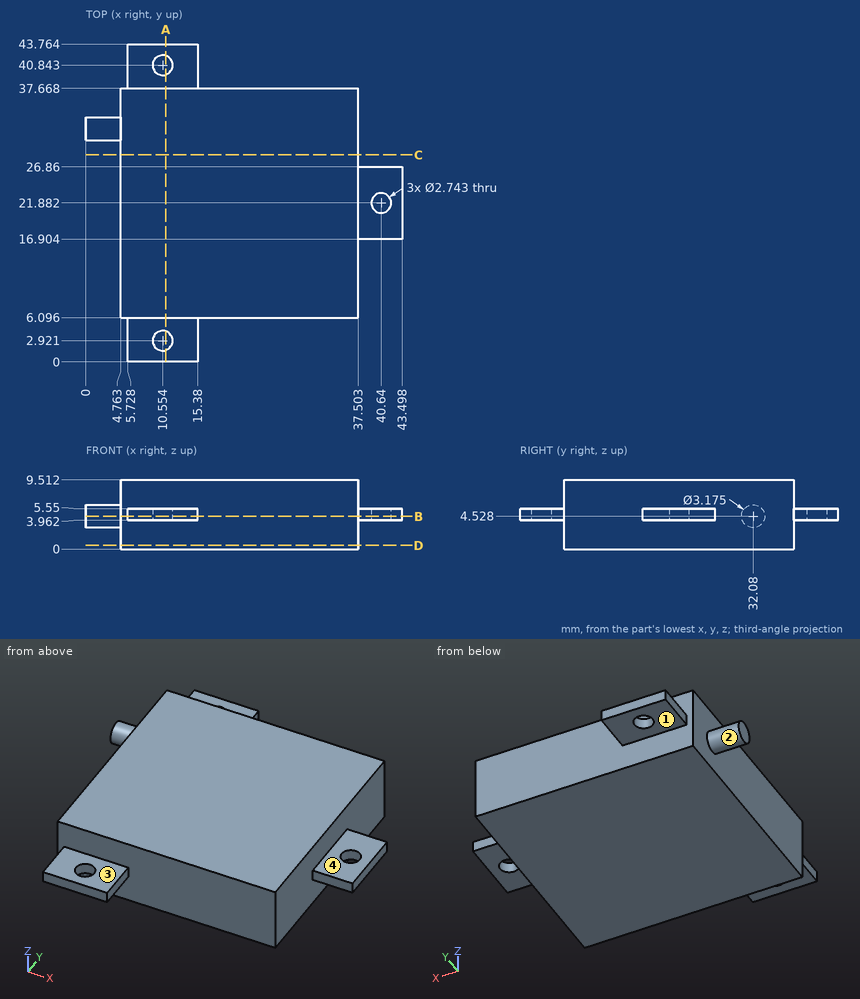
For this review, use the dimensioned drawing (mm, ordinates from the lowest corner) and the shaded views. A direction names the side the tool comes from. Round coordinates to 2 decimals unless told otherwise and drop trailing zeros. Order: outer loops, then holes, each group sorted by start corner. A loop starts at its lowest first (then second) coordinate and runs counter-clockwise, first axis right, second up. Notation, with made-up numbers: M 4,56.25 L 36,56.25 A15 cw 36,80.25 Z; hole C -16,82 d9. An arc over 180 degrees is marked long. Use a Markdown table: item, result. Add a question column.
Item 1: Add section B-B, the plane z = 4.5. Give the boundary of the cut face in (x, y) (1 decimal), then the cut area to 3 significant figures.
Item 2: Tool access review of the marked faces 1, 2, 3 and 4: name each direction out of +Z, -Z, +X, -X, +Y, -Y from which nothing blocks a thin tool from reaching the whole face with its end or side.
Item 3: Insertion check: pin 1 (4 mm diameter, centred on x = 19.5, z = 7, fed in from +Y); pin 2 (6.5 mm diameter, centred on x = 40, y = 21.5, fed in from +Z); pin 3 (5 mm diameter, centred on y = 19, z = 6, fed in from -X); pin 4 (5 mm diameter, centred on x = 8.5, y = 2, fed in from -Z). Each pin has a flat end and moves straight along its axis. Give the tip position at first contact, or say it passes through.
Item 4: Add section D-D, the plane z = 0.5. Give the boundary of the cut face in (x, y) (1 decimal).
Item 5: Add section C-C, the plane y = 28.5. Give the boundary of the cut face in (x, z).
Item 6: Add section A-A, the plane x = 11. State how many separate pieces and enclosed holes the cut face has.
Item 7: To check wall thickness, follow line 1 along Y through (x, z) = (32, 7.75) (1 decimal); line 2 along X through (y, z) = (30, 7.75); line 3 along X through (y, z) = (18, 5.25). State the ranges of each line that lie inside material, in increasing order.
Geometry results:
| question | item | result |
|---|---|---|
| 1 | outline | M 0,30.5 L 4.8,30.5 L 4.8,6.1 L 5.7,6.1 L 5.7,0 L 15.4,0 L 15.4,6.1 L 37.5,6.1 L 37.5,16.9 L 43.5,16.9 L 43.5,26.9 L 37.5,26.9 L 37.5,37.7 L 15.4,37.7 L 15.4,43.8 L 5.7,43.8 L 5.7,37.7 L 4.8,37.7 L 4.8,33.7 L 0,33.7 Z; hole C 10.6,2.9 d2.7; hole C 10.6,40.8 d2.7; hole C 40.6,21.9 d2.7 |
| 1 | area | 1,210 mm² |
| 2 | face 1 | -Z, +X, -X, +Y |
| 2 | face 2 | -X |
| 2 | face 3 | +Z, +X, -X, -Y |
| 2 | face 4 | +Z, +X, +Y, -Y |
| 3 | pin 1 | stops at y = 37.67 |
| 3 | pin 2 | stops at z = 9.51 |
| 3 | pin 3 | stops at x = 4.76 |
| 3 | pin 4 | stops at z = 3.96 |
| 4 | outline | M 4.8,6.1 L 37.5,6.1 L 37.5,37.7 L 4.8,37.7 Z |
| 5 | outline | M 4.76,0 L 37.5,0 L 37.5,9.51 L 4.76,9.51 Z |
| 6 | separate pieces | 3 |
| 6 | enclosed holes | 0 |
| 7 | line 1 | y = 6.1 to 37.7 |
| 7 | line 2 | x = 4.76 to 37.5 |
| 7 | line 3 | x = 4.76 to 43.5 |
